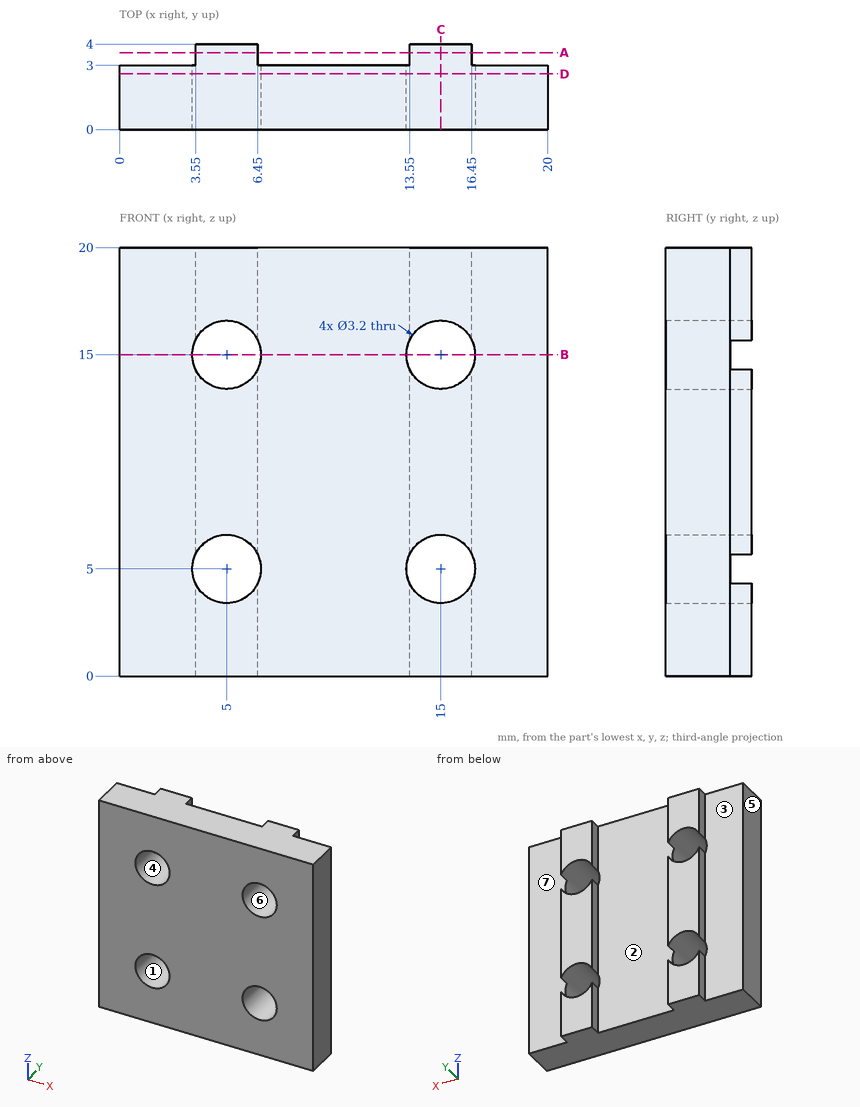
Print and shaded views of the part. All mm, measured from the part's lowest x, y and z. A direction names the side the tool comes from. Coordinates: 2 decimals unless noted, no trailing zeros. Loops run counter-clockwise (first coordinate to the right, second up) from the corner with the lowest first, then second, coordinate; pieces in that order, holes last. Notation, with made-up numbers: (4, -16) - (21, -16) arc R4 cw to (21, -11) - close; hole circle Ø2 at (75, 11.25). An arc over 180 degrees is marked (long way). Use one line per item in the form item = value. Start each with the question number.
1) Band-saw the part on D-D (y = 2.6). Give the cut face in (x, z), and give its area (3 significant figures).
2) Band-saw the part on C-C (x = 15). Give the cut face in (y, z).
3) Tool access for the marked faces 1, 2 and 3: list every direction of +Z, -Z, +X, -X, +Y, -Y with a clear straight run to the whole face (end or side of a thin tool).
4) Drill centre lines: L1, parallel to Z at x = 5, y = 1; L2, parallel to X at y = 1.6, z = 15.5. Where is each one in solid material? Low to high. Write a range as from..to.
5) Two-plate mould, pull along X, no slides. Class the marked faces 4, 5, 6 and 7: +X half, -X half, draft (parallel to the pull), parting line (faces both ways), or undercut.
6) Band-saw the part on B-B (z = 15). Give the cut face in (x, y).
7) Flat gauge pins, fed straight in: pin 1 (0.8 mm diameter, centred on y = 3.5, z = 2.5, fed in from -X); pin 2 (2 mm diameter, centred on x = 11.5, z = 9.5, fed in from +Y); pin 3 (0.5 mm diameter, centred on y = 3.5, z = 9.5, fed in from +X). Where does each tip first touch, or does it go through?
8) Band-saw the part on A-A (y = 3.6). Give the cut face in (x, z), and give its area (3 significant figures).
Check values:
q1.outline = (0, 0) - (20, 0) - (20, 20) - (0, 20) - close; hole circle Ø3.2 at (5, 5); hole circle Ø3.2 at (5, 15); hole circle Ø3.2 at (15, 5); hole circle Ø3.2 at (15, 15)
q1.area = 368 mm2
q2.outline = (0, 0) - (4, 0) - (4, 3.4) - (0, 3.4) - close; (0, 6.6) - (4, 6.6) - (4, 13.4) - (0, 13.4) - close; (0, 16.6) - (4, 16.6) - (4, 20) - (0, 20) - close
q3.face_1 = +Y, -Y
q3.face_2 = +Z, -Z, +Y
q3.face_3 = +Z, -Z, -X, +Y
q4.L1 = 0..3.4, 6.6..13.4, 16.6..20
q4.L2 = 0..3.48, 6.52..13.48, 16.52..20
q5.face_4 = undercut
q5.face_5 = -X half
q5.face_6 = undercut
q5.face_7 = draft
q6.outline = (0, 0) - (3.4, 0) - (3.4, 3) - (0, 3) - close; (6.6, 0) - (13.4, 0) - (13.4, 3) - (6.6, 3) - close; (16.6, 0) - (20, 0) - (20, 3) - (16.6, 3) - close
q7.pin_1 = 3.55
q7.pin_2 = 3
q7.pin_3 = 16.45
q8.outline = (3.55, 0) - (6.45, 0) - (6.45, 4.32) arc R1.6 cw to (3.55, 4.32) - close; (3.55, 5.68) arc R1.6 cw to (6.45, 5.68) - (6.45, 14.32) arc R1.6 cw to (3.55, 14.32) - close; (3.55, 15.68) arc R1.6 cw to (6.45, 15.68) - (6.45, 20) - (3.55, 20) - close; (13.55, 0) - (16.45, 0) - (16.45, 4.32) arc R1.6 cw to (13.55, 4.32) - close; (13.55, 5.68) arc R1.6 cw to (16.45, 5.68) - (16.45, 14.32) arc R1.6 cw to (13.55, 14.32) - close; (13.55, 15.68) arc R1.6 cw to (16.45, 15.68) - (16.45, 20) - (13.55, 20) - close
q8.area = 84.9 mm2
